Part model, mm, in its own coordinate system. Face numbers are marked on the shaded views. A direction names the side the tool comes from. Give positions to 0.01 mm unless a question says otherwise; leave off trailing zeros. Order: outer loops, then holes, each group sorted by start corner. A loop starts at its lowest first (then second) coordinate and runs counter-clockwise, first axis right, second up. Notation, with made-up numbers: (1, -10) - (30, -10) arc R20 cw to (30, 29) - close; hole circle Ø10 at (89, 52.5). An arc over 180 degrees is marked (long way). Use one line per item in the form item = value. Start each with the question number.
1. Drill centre lines: line 1 (X direction, y = 8.5, z = -7); line 2 (Y direction, x = -10.75, z = -3); line 3 (X direction, y = -12, z = -6.75). Where is each one in solid material? Low to high.
2. Band-saw the part on C-C, the plane x = -2.5. List the corners of the cut face in (y, z), plus the area to 3 significant figures.
3. Band-saw the part on B-B, the plane z = -5.75. List the corners of the cut face in (x, y).
4. Band-saw the part on D-D, the plane y = 4.75. List the corners of the cut face in (x, z), plus the area to 3 significant figures.
5. Tool access for the marked faces 1 and 2: list every direction of +Z, -Z, +X, -X, +Y, -Y with a clear straight run to the whole face (end or side of a thin tool).
6. Pin check, flat tips, straight feed: P1, Ø1.5, axis at x = 0, z = -1.5, coming from the +Y side; P2, Ø1, axis at x = -4.5, z = -2.5, coming from the +Y side; P3, Ø1, axis at y = 2.5, z = -1, coming from the +X side. Stop position of each tip, or through.
7. Band-saw the part on A-A, the plane x = 1.5. List the corners of the cut face in (y, z).
8. Pull direction X, two halves, no side cores. Call the marked faces 3 and 4: +X half, -X half, draft (parallel to the pull), parting line (faces both ways), or undercut.
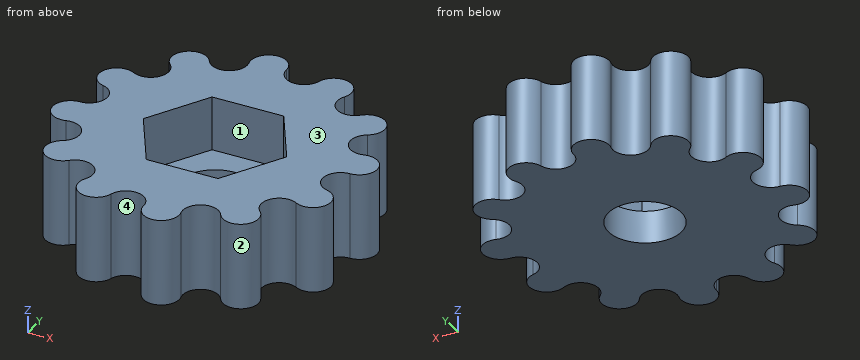
Autodesk Inventor part; units mm, degrees
ref_plane "YZ Plane" through (0, 0, 0) normal (1, 0, 0) x (0, 1, 0)
ref_plane "XZ Plane" through (0, 0, 0) normal (0, 1, 0) x (-1, 0, 0)
ref_plane "XY Plane" through (0, 0, 0) normal (0, 0, 1) x (1, 0, 0)
sketch "Sketch1" plane through (0, 0, 0) normal (0, 0, 1) x (1, 0, 0)
  line L0 (3.3198, 5.75) -> (6.6395, 0)
  line L1 (6.6395, 0) -> (3.3198, -5.75)
  line L2 (3.3198, -5.75) -> (-3.3198, -5.75)
  line L3 (-3.3198, -5.75) -> (-6.6395, 0)
  line L4 (-6.6395, 0) -> (-3.3198, 5.75)
  line L5 (-3.3198, 5.75) -> (3.3198, 5.75)
  circle A0 centre (0, 0) radius 12.5
  dimension "d0" = 11.5
  dimension "d1" = 25
extrude "Extrusion1" add sketch "Sketch1" against normal blind 5
sketch "Sketch2" plane through (0, 0, -5) normal (0, 0, -1) x (-1, 0, 0)
  circle A0 centre (0, 0) radius 12.5
extrude "Extrusion2" add sketch "Sketch2" along normal blind 3
sketch "Sketch3" plane through (0, 0, -8) normal (0, 0, -1) x (-1, 0, 0)
  circle A0 centre (0, 0) radius 12.5 construction
hole "Hole1" at (0, 0, -8) direction (0, 0, 1) diameter 6.756 end through all
sketch "Sketch4" plane through (0, 0, 0) normal (0, 0, 1) x (1, 0, 0)
  circle A0 centre (0, 0) radius 12.5
  arc A1 (0, 12.5) -> (3.2352, 12.0741) centre (1.6457, 12.5) ccw
  arc A2 (6.25, 10.8253) -> (3.2352, 12.0741) centre (4.8248, 11.6481) ccw
  line L0 (0, 12.5) -> (0, 0) construction
  line L1 (-6.25, 10.8253) -> (0, 0) construction
  line L2 (-10.8253, 6.25) -> (0, 0) construction
  line L3 (-12.5, 0) -> (0, 0) construction
  line L4 (-10.8253, -6.25) -> (0, 0) construction
  line L5 (-6.25, -10.8253) -> (0, 0) construction
  line L6 (0, -12.5) -> (0, 0) construction
  line L7 (6.25, -10.8253) -> (0, 0) construction
  line L8 (10.8253, -6.25) -> (0, 0) construction
  line L9 (12.5, 0) -> (0, 0) construction
  line L10 (10.8253, 6.25) -> (0, 0) construction
  line L11 (6.25, 10.8253) -> (0, 0) construction
  dimension "d15" = 360
extrude "Extrusion3" cut sketch "Sketch4" against normal through all contours A0 A1 picked at (1.5636, 11.877)
extrude "Extrusion4" add sketch "Sketch4" against normal up to surface (8 mm away) contours A0 A2
pattern_circular "Circular Pattern1" count 12 over 360 about axis through (0, 0, -10) along (0, 0, 1) of "Extrusion3", "Extrusion4"
properties part number "knurled nut"
From the geometry:
q1.line_1 = -8.58 to 7, 8.35 to 11.43
q1.line_2 = -9.14 to -6.2, -3.45 to 6.21
q1.line_3 = -6.43 to -3.21, -0.08 to 3.22
q2.outline = (-11.09, -8) - (-2.27, -8) - (-2.27, -5) - (-5.75, -5) - (-5.75, 0) - (-11.09, 0) - close; (2.27, -8) - (13.91, -8) - (13.91, 0) - (5.75, 0) - (5.75, -5) - (2.27, -5) - close
q2.area = 129 mm²
q3.outline = (-12.5, 0) arc R1.65 ccw (long way) to (-12.07, -3.24) arc R1.65 cw to (-10.83, -6.25) arc R1.65 ccw (long way) to (-8.84, -8.84) arc R1.65 cw to (-6.25, -10.83) arc R1.65 ccw (long way) to (-3.24, -12.07) arc R1.65 cw to (0, -12.5) arc R1.65 ccw (long way) to (3.24, -12.07) arc R1.65 cw to (6.25, -10.83) arc R1.65 ccw (long way) to (8.84, -8.84) arc R1.65 cw to (10.83, -6.25) arc R1.65 ccw (long way) to (12.07, -3.24) arc R1.65 cw to (12.5, 0) arc R1.65 ccw (long way) to (12.07, 3.24) arc R1.65 cw to (10.83, 6.25) arc R1.65 ccw (long way) to (8.84, 8.84) arc R1.65 cw to (6.25, 10.83) arc R1.65 ccw (long way) to (3.24, 12.07) arc R1.65 cw to (0, 12.5) arc R1.65 ccw (long way) to (-3.24, 12.07) arc R1.65 cw to (-6.25, 10.83) arc R1.65 ccw (long way) to (-8.84, 8.84) arc R1.65 cw to (-10.83, 6.25) arc R1.65 ccw (long way) to (-12.07, 3.24) arc R1.65 cw to start; hole circle Ø6.76 at (0, 0)
q4.outline = (-13.29, -8) - (10, -8) - (10, 0) - (3.9, 0) - (3.9, -5) - (-3.9, -5) - (-3.9, 0) - (-13.29, 0) - close
q4.area = 147 mm²
q5.face_1 = +Z
q5.face_2 = +Z, -Z
q6.P1 = 13.88
q6.P2 = 10.22
q6.P3 = 14.11
q7.outline = (-14.14, -8) - (-3.03, -8) - (-3.03, -5) - (-5.75, -5) - (-5.75, 0) - (-14.14, 0) - close; (3.03, -8) - (10.86, -8) - (10.86, 0) - (5.75, 0) - (5.75, -5) - (3.03, -5) - close
q8.face_3 = draft
q8.face_4 = undercut
